from build123d import *


with BuildPart() as part:
    # Sketch12 → Revolve2 (revolve)
    with BuildSketch(Plane(origin=(0, 0, 0), x_dir=(0, 0, -1), z_dir=(1, 0, 0))):
        Polygon((996.979831822, 0), (996.979831822, 448.154362623), (1015.309498351, 448.154362623), (1015.309498351, 460.844131759), (1035.049139229, 460.844131759), (1035.049139229, 448.154362623), (1035.049139229, 438.418962309), (1049.739382804, 438.418962309), (1049.739382804, 107.862695979), (1082.4718279, 107.862695979), (1082.4718279, 93.31637014), (1090.933076859, 84.855121181), (1156.280143072, 84.855121181), (1156.280143072, 76.411453441), (1617.589293356, 80.633287311), (1630.272376185, 93.31637014), (1688.665257097, 93.31637014), (1688.665257097, 62.954107013), (1898.216315919, 62.954107013), (1910.575471981, 50.594950951), (1922.934628043, 62.954107013), (1950.934428364, 62.954107013), (1963.792504571, 62.954107013), (1963.792504571, 116.171139603), (1963.792504571, 128.530295665), (1976.151660632, 128.530295665), (1976.151660632, 93.31637014), (1983.424823552, 100.58953306), (1983.424823552, 35.664179648), (3155.097212513, 35.664179648), (3163.146026729, 43.712993865), (3194.167030322, 43.712993865), (3202.215844538, 35.664179648), (3212.399611966, 35.664179648), (3236.709720825, 50.594950951), (3236.709720825, 0), align=None)
    revolve(axis=Axis((0, 0, 0), (0, 0, -1)))


solid = part.part
Here's how the part is built. I have some questions about the finished solid (model axes, mm). A direction names the side the tool comes from. Give positions to 0.01 mm unless a question says otherwise; leave off trailing zeros. Order: outer loops, then holes, each group sorted by start corner. A loop starts at its lowest first (then second) coordinate and runs counter-clockwise, first axis right, second up. Notation, with made-up numbers: M -19,25.25 L 31,25.25 A17 ccw 31,37.25 Z; hole C 56.5,12.5 d3. An arc over 180 degrees is marked long. Answer as a JSON object with one key per item and string values. Group by question number.
1) Suppose I cut it at C-C, the plane z = -2537.5. Write out the boundary of the cut face in (x, y).
2) Suppose I cut it at A-A, the plane y = -323.5. Write out the boundary of the cut face in (x, z), plus the area to 3 significant figures.
3) I'm going to push a flat-ended pin straight in: pin 1 Ø6 at (x, y) = (-274, 232) entering from -Z. Where does the tip first touch, or does it pass through?
4) We'd pull the mould along Z, two halves only. Please class faces 1 (the flat face through (-442, -100, -1015.309)), 2 (the flat face through (67, 66, -1976.152)), 3 (the flat face through (1, -1, -3236.71)): pulls with the +Z half, pulls with the -Z half, needs draft (parallel to the pull), parting line crosses it, or undercut.
5) Suppose I cut it at D-D, the plane z = -1435. Write out the boundary of the cut face in (x, y).
6) On a 3-axis mill with a long thin cutter (end or side, diameter ignored), from which of +Z, -Z, +X, -X, +Y, -Y can I reach the whole of each face in a straight line? I mean faces 4 (the cylindrical face through (-42.674, -9.476, -3178.874)), 5 (the flat face through (-169, -407, -1035.049)), 6 (the cylindrical face through (-408.85, 212.65, -1025.32)). Say none if no direction works.
7) Suppose I cut it at B-B, the plane x = 212. Write out the boundary of the cut face in (y, z), plus the area to 3 significant figures.
8) Please list where these lines run through material, in increasing order: L1, parallel to Z at x = -153, y = -204.5; L2, parallel to Z at x = 37.5, y = 47.5; L3, parallel to X at y = 56, z = -1856.5. Write a range as [from, to].
Results found:
{
 "1": {"outline": "C 0,0 d71.33"},
 "2": {"outline": "M -328.21,-1035.05 L -295.9,-1035.05 L -295.9,-1049.74 L 295.9,-1049.74 L 295.9,-1035.05 L 328.21,-1035.05 L 328.21,-1015.31 L 310.15,-1015.31 L 310.15,-996.98 L -310.15,-996.98 L -310.15,-1015.31 L -328.21,-1015.31 Z", "area": "33,000 mm²"},
 "3": {"pin 1": "z = -1049.74"},
 "4": {"face 1": "pulls with the +Z half", "face 2": "undercut", "face 3": "pulls with the -Z half"},
 "5": {"outline": "C 0,0 d157.92"},
 "6": {"face 4": "none", "face 5": "-Z", "face 6": "+Z, -Z"},
 "7": {"outline": "M -409.19,-1035.05 L -383.75,-1035.05 L -383.75,-1049.74 L 383.75,-1049.74 L 383.75,-1035.05 L 409.19,-1035.05 L 409.19,-1015.31 L 394.84,-1015.31 L 394.84,-996.98 L -394.84,-996.98 L -394.84,-1015.31 L -409.19,-1015.31 Z", "area": "41,900 mm²"},
 "8": {"L1": "[-1049.74, -996.98]", "L2": "[-1983.42, -1920.5], [-1900.65, -996.98]", "L3": "[-28.76, 28.76]"}
}
